Read the model definition and answer for the solid it produces. Units are mm, in the model's axes. Face numbers are marked on the shaded views. Coordinates: 2 decimals unless noted, no trailing zeros. Use one line per item in the form item = value. Start each with the question number.
1. Flat-ended cylindrical pins translate along their axes: pin 1 (2.5 mm diameter, centred on x = 33.06, z = -33.06, fed in from -Y); pin 2 (12 mm diameter, centred on x = -8, z = 35, fed in from +Y). Find the tip coordinate at first contact, or state that the pin passes through.
2. Find the intervals of material crossed by probe 1 along Z at (x, y) = (0, 2.6); probe 2 along X at (y, z) = (6.25, -70); probe 3 along Z at (x, y) = (65, 4.25), in increasing order. Write a range as [from, to].
3. For a pull along X with two mould halves and no side action, classify the marked faces 1 and 2 as released by +X, released by -X, zero draft, split by the parting line, or undercut.
4. The part is cut by section A-A (y = 3.25). Give the number of separate pieces and of enclosed holes in the cut face, plus the area to 3 significant figures.
from build123d import *

# Parameters (mm, degrees)
SKETCH1_W           = 200
SKETCH1_H           = 150
SKETCH1_R           = 55
SKETCH1_R_2         = 2
BOSS_EXTRUDE1_DEPTH = 10
SKETCH1_3_R         = 55
SKETCH1_3_R_2       = 38.5
BOSS_EXTRUDE2_DEPTH = 5
SKETCH1_4_R         = 38.5
BOSS_EXTRUDE3_DEPTH = 9
SKETCH2_R           = 2
CUT_EXTRUDE1_DEPTH  = 6
SKETCH1_5_R         = 38.5
CUT_EXTRUDE2_DEPTH  = 11
CUT_EXTRUDE3_DEPTH  = 11
CHAMFER1_SIZE       = 0.1


with BuildPart() as part:
    # Sketch1 → Boss-Extrude1 (new body)
    with BuildSketch(Plane(origin=(0, 0, 0), x_dir=(1, 0, 0), z_dir=(0, 1, 0))):
        with Locations((-25, 0)):
            Rectangle(SKETCH1_W, SKETCH1_H)
        Circle(SKETCH1_R, mode=Mode.SUBTRACT)
        with Locations((65, 70)):
            Circle(SKETCH1_R_2, mode=Mode.SUBTRACT)
        with Locations((-115, 70)):
            Circle(SKETCH1_R_2, mode=Mode.SUBTRACT)
        with Locations((65, -70)):
            Circle(SKETCH1_R_2, mode=Mode.SUBTRACT)
        with Locations((-115, -70)):
            Circle(SKETCH1_R_2, mode=Mode.SUBTRACT)
        with Locations((-25, 70)):
            Circle(SKETCH1_R_2, mode=Mode.SUBTRACT)
        with Locations((-25, -70)):
            Circle(SKETCH1_R_2, mode=Mode.SUBTRACT)
        with Locations((65, 0)):
            Circle(SKETCH1_R_2, mode=Mode.SUBTRACT)
        with Locations((-115, 0)):
            Circle(SKETCH1_R_2, mode=Mode.SUBTRACT)
    extrude(amount=BOSS_EXTRUDE1_DEPTH)

    # Sketch1_3 → Boss-Extrude2 (add)
    with BuildSketch(Plane(origin=(0, 0, 0), x_dir=(1, 0, 0), z_dir=(0, 1, 0))):
        Circle(SKETCH1_3_R)
        Circle(SKETCH1_3_R_2, mode=Mode.SUBTRACT)
    extrude(amount=BOSS_EXTRUDE2_DEPTH)

    # Sketch1_4 → Boss-Extrude3 (add)
    with BuildSketch(Plane(origin=(0, 0, 0), x_dir=(1, 0, 0), z_dir=(0, 1, 0))):
        Circle(SKETCH1_4_R)
    extrude(amount=BOSS_EXTRUDE3_DEPTH)

    # Sketch2 → Cut-Extrude1 (cut, through all)
    with BuildSketch(Plane(origin=(0, 5, 0), x_dir=(1, 0, 0), z_dir=(0, 1, 0))):
        with Locations((0, 46.75)):
            Circle(SKETCH2_R)
        with Locations((33.05724202, 33.05724202)):
            Circle(SKETCH2_R)
        with Locations((46.75, 0)):
            Circle(SKETCH2_R)
        with Locations((33.05724202, -33.05724202)):
            Circle(SKETCH2_R)
        with Locations((0, -46.75)):
            Circle(SKETCH2_R)
        with Locations((-33.05724202, -33.05724202)):
            Circle(SKETCH2_R)
        with Locations((-46.75, 0)):
            Circle(SKETCH2_R)
        with Locations((-33.05724202, 33.05724202)):
            Circle(SKETCH2_R)
    extrude(amount=-CUT_EXTRUDE1_DEPTH, mode=Mode.SUBTRACT)

    # Sketch1_5 → Cut-Extrude2 (cut, through all)
    with BuildSketch(Plane(origin=(0, 0, 0), x_dir=(1, 0, 0), z_dir=(0, 1, 0))):
        Circle(SKETCH1_5_R)
    extrude(amount=CUT_EXTRUDE2_DEPTH, mode=Mode.SUBTRACT)

    # Sketch4 → Cut-Extrude3 (cut, through all)
    with BuildSketch(Plane(origin=(0, 10, 0), x_dir=(1, 0, 0), z_dir=(0, 1, 0))):
        with BuildLine():
            Line((-61, 30), (-61, 20))
            ThreePointArc((-61, 20), (-65, 16), (-69, 20))
            Line((-69, 20), (-69, 30))
            ThreePointArc((-69, 30), (-65, 34), (-61, 30))
        make_face()
        with BuildLine():
            Line((-74, -25), (-74, -15))
            ThreePointArc((-74, -15), (-70, -11), (-66, -15))
            Line((-66, -15), (-66, -25))
            ThreePointArc((-66, -25), (-70, -29), (-74, -25))
        make_face()
    extrude(amount=-CUT_EXTRUDE3_DEPTH, mode=Mode.SUBTRACT)

    # Chamfer1
    chamfer1_edges = [part.edges().sort_by_distance(p)[0] for p in [
        (-65, 0, -34),
        (-61, 0, -25),
        (-65, 0, -16),
        (-69, 0, -25),
        (-65, 10, -34),
        (-69, 10, -25),
        (-65, 10, -16),
        (-61, 10, -25),
        (-70, 0, 29),
        (-74, 0, 20),
        (-70, 0, 11),
        (-66, 0, 20),
        (-70, 10, 29),
        (-66, 10, 20),
        (-70, 10, 11),
        (-74, 10, 20),
        (-117, 10, 0),
        (-27, 0, 70),
        (-27, 0, -70),
        (63, 0, 70),
        (-117, 0, -70),
        (63, 0, -70),
        (-25, 0, 75),
        (63, 10, 0),
        (-125, 0, 0),
        (-25, 0, -75),
        (75, 0, 0),
        (-117, 0, 70),
        (63, 0, 0),
        (-117, 0, 0),
        (-117, 10, 70),
        (75, 10, 0),
        (-25, 10, -75),
        (-55, 5, 0),
        (-125, 10, 0),
        (-25, 10, 75),
        (-55, 10, 0),
        (63, 10, -70),
        (-117, 10, -70),
        (-2, 0, -46.75),
        (-2, 5, -46.75),
        (63, 10, 70),
        (31.05724202, 0, -33.05724202),
        (31.05724202, 5, -33.05724202),
        (44.75, 0, 0),
        (44.75, 5, 0),
        (31.05724202, 0, 33.05724202),
        (31.05724202, 5, 33.05724202),
        (-27, 10, -70),
        (-2, 0, 46.75),
        (-2, 5, 46.75),
        (-35.05724202, 0, 33.05724202),
        (-35.05724202, 5, 33.05724202),
        (-48.75, 0, 0),
        (-48.75, 5, 0),
        (-27, 10, 70),
        (-35.05724202, 0, -33.05724202),
        (-35.05724202, 5, -33.05724202),
        (-38.5, 5, 0),
        (-38.5, 0, 0),
    ]]
    chamfer(chamfer1_edges, length=CHAMFER1_SIZE)


solid = part.part
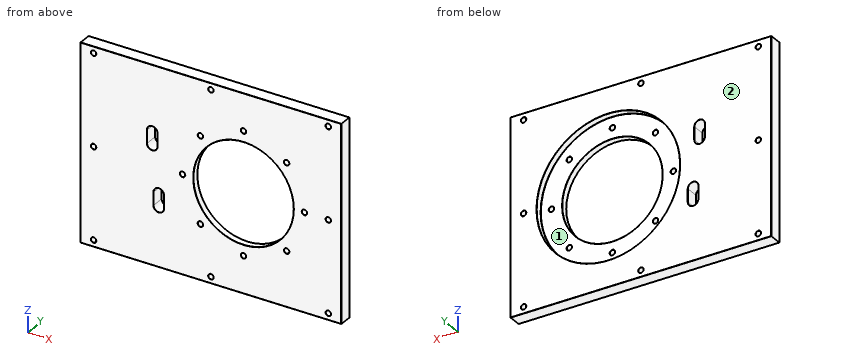
Computed values:
q1.pin_1 = through
q1.pin_2 = 5
q2.probe_1 = [-75, -48.75], [-44.75, -38.5], [38.5, 44.75], [48.75, 75]
q2.probe_2 = [-125, -117], [-113, -27], [-23, 63], [67, 75]
q2.probe_3 = [-75, -72], [-68, -2], [2, 68], [72, 75]
q3.face_1 = undercut
q3.face_2 = zero draft
q4.separate_pieces = 1
q4.enclosed_holes = 19
q4.area = 24,900 mm²
